```python
from build123d import *

# Parameters (mm, degrees)
F0_W         = 152.4
F0_H         = 44.45
F1_DEPTH     = 2
F2_W         = 152.4
F2_H         = 6.35
F3_DEPTH     = 18.796
F4_R         = 1.75
F5_DEPTH     = 25
F7_DEPTH     = 25.401
F8_SIZE      = 1.8
F9_T4_DEPTH  = 152.4
F9_S5_R      = 9
F9_T6_DEPTH  = 78
F9_T10_DEPTH = 152.4
F9_S11_R     = 9
F9_T12_DEPTH = 78
F10_R        = 2


# Not quite as in the source:
# - a fillet or chamfer that OpenCascade refuses, or shapes differently, is made with other operations: its cross-section is extruded or revolved along the edge and cut away or added
# - a feature names something its author has since deleted; it is built from what else it names


with BuildPart() as f1:
    # F0 (on Top) → F1 (new body)
    with BuildSketch(Plane.XY):
        Rectangle(F0_W, F0_H)
    extrude(amount=F1_DEPTH)

    # F2 (on face) → F3 (join)
    with BuildSketch(Plane(origin=(0, 0, 0), x_dir=(1, 0, 0), z_dir=(0, 0, -1))):
        Rectangle(F2_W, F2_H)
    extrude(amount=F3_DEPTH)

    # F4 (on face) → F5 (cut)
    with BuildSketch(Plane(origin=(0, 0, 0), x_dir=(1, 0, 0), z_dir=(0, 0, -1))):
        with Locations((48, -12.7)):
            Circle(F4_R)
        with Locations((-48, -12.7)):
            Circle(F4_R)
        with Locations((-48, 12.7)):
            Circle(F4_R)
        with Locations((48, 12.7)):
            Circle(F4_R)
    extrude(amount=-F5_DEPTH, mode=Mode.SUBTRACT)

    # F6 (on face) → F7 (cut, through all)
    with BuildSketch(Plane(origin=(0, 3.175, 0), x_dir=(-1, 0, 0), z_dir=(0, 1, 0))):
        with BuildLine():
            ThreePointArc((-9, -9.398), (0, -18.398), (9, -9.398))
            ThreePointArc((9, -9.398), (0, -0.398), (-9, -9.398))
        make_face()
        with BuildLine():
            Line((9, -18.796), (9, -9.398))
            ThreePointArc((9, -9.398), (0, -18.398), (-9, -9.398))
            Line((-9, -9.398), (-9, -18.796))
            Line((-9, -18.796), (9, -18.796))
        make_face()
    extrude(amount=-F7_DEPTH, mode=Mode.SUBTRACT)

    # F8
    f8_edges = [f1.edges().sort_by_distance(p)[0] for p in [
        (46.25, -12.7, 2),
        (-49.75, -12.7, 2),
        (-49.75, 12.7, 2),
        (46.25, 12.7, 2),
    ]]
    chamfer(f8_edges, length=F8_SIZE)

    # F9: chamfer of 1 on 2 edges, made by hand


with BuildPart() as f9_tool2:
    # F9_s3 → F9_t4 (new body)
    with BuildSketch(Plane.YZ.offset(-76.2)):
        Polygon((3.175, -1), (4.175, 0), (3.175, 0), align=None)
    extrude(amount=F9_T4_DEPTH)

    # F9_s5 → F9_t6 (cut, symmetric)
    with BuildSketch(Plane.XZ.offset(-3.7)):
        with Locations((0, -9.398)):
            Circle(F9_S5_R)
    extrude(amount=F9_T6_DEPTH, both=True, mode=Mode.SUBTRACT)


with BuildPart() as f1_1:
    add(f1.part)

    # F9_t1: union F9_tool2
    add(f9_tool2.part)


with BuildPart() as f9_tool8:
    # F9_s9 → F9_t10 (new body)
    with BuildSketch(Plane.YZ.offset(76.2)):
        Polygon((-4.175, 0), (-3.175, -1), (-3.175, 0), align=None)
    extrude(amount=-F9_T10_DEPTH)

    # F9_s11 → F9_t12 (cut, symmetric)
    with BuildSketch(Plane.XZ.offset(3.7)):
        with Locations((0, -9.398)):
            Circle(F9_S11_R)
    extrude(amount=F9_T12_DEPTH, both=True, mode=Mode.SUBTRACT)


with BuildPart() as f1_2:
    add(f1_1.part)

    # F9_t7: union F9_tool8
    add(f9_tool8.part)

    # F10
    f10_edges = [f1_2.edges().sort_by_distance(p)[0] for p in [
        (9, 0, -18.796),
        (-9, 0, -18.796),
    ]]
    fillet(f10_edges, radius=F10_R)


solid = f1_2.part
```
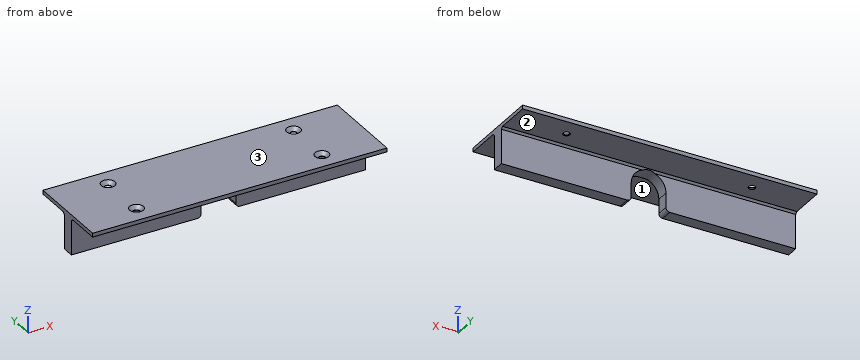
The model under review builds one solid part; all positions refer to its coordinate system, in mm. Face numbers are marked on the shaded views. A direction names the side the tool comes from. Coordinates: 2 decimals unless noted, no trailing zeros. Loops run counter-clockwise (first coordinate to the right, second up) from the corner with the lowest first, then second, coordinate; pieces in that order, holes last. Notation, with made-up numbers: (59, 61) -> (79, 61) arc R18 ccw to (79, 83) -> close; hole circle Ø6 at (70, 70). An arc over 180 degrees is marked (long way). Answer as CSV lines item,"result".
Item 1: Take a section at B-B, the plane z = -12.75. State the section outline as (x, y) points (3 decimals).
Results below:
outline,"(-76.2, -3.175) -> (-9, -3.175) -> (-9, 3.175) -> (-76.2, 3.175) -> close; (9, -3.175) -> (76.2, -3.175) -> (76.2, 3.175) -> (9, 3.175) -> close"
Item 2: Take a section at D-D, the plane x = 0. State the section outline as (y, z) points (3 decimals).
Results below:
outline,"(-22.225, 0) -> (-4.175, 0) -> (-3.777, -0.398) -> (3.777, -0.398) -> (4.175, 0) -> (22.225, 0) -> (22.225, 2) -> (-22.225, 2) -> close"
Item 3: Take a section at A-A, the plane x = 48. State the section outline as (y, z) points (3 decimals), and give its area (3 significant figures).
Results below:
outline,"(-22.225, 0) -> (-14.45, 0) -> (-14.45, 0.2) -> (-16.25, 2) -> (-22.225, 2) -> close; (-10.95, 0) -> (-4.175, 0) -> (-3.175, -1) -> (-3.175, -18.796) -> (3.175, -18.796) -> (3.175, -1) -> (4.175, 0) -> (10.95, 0) -> (10.95, 0.2) -> (9.15, 2) -> (-9.15, 2) -> (-10.95, 0.2) -> close; (14.45, 0) -> (22.225, 0) -> (22.225, 2) -> (16.25, 2) -> (14.45, 0.2) -> close"
area,"189 mm2"
Item 4: Insertion check: pin 1 (12 mm diameter, centred on x = -13, z = -11.5, fed in from -Y) (3 decimals); pin 2 (10 mm diameter, centred on x = -16.5, z = -7.5, fed in from +Y) (3 decimals); pin 3 (3 mm diameter, centred on x = -48, y = 12.7, fed in from -Z); pin 4 (5.5 mm diameter, centred on x = 17, y = 13.5, fed in from -Z). Each pin has a flat end and moves straight along its axis. Give the tip position at first contact, or say it passes through.
Results below:
pin 1,"stops at y = -3.175"
pin 2,"stops at y = 3.175"
pin 3,"passes through"
pin 4,"stops at z = 0"
Item 5: Machinability: for the marked faces 1, 2 and 3, which of the approach directions +Z, -Z, +X, -X, +Y, -Y give a long, thin tool a straight path to every point of the face, cutting with its end or side? Answer none if there is none.
Results below:
face 1,"-Z, +X, -X, -Y"
face 2,"-Z, +X, -X, +Y"
face 3,"+Z, +X, -X, +Y, -Y"
Item 6: Take a section at C-C, the plane y = 12.7. State the section outline as (x, z) points.
Results below:
outline,"(-76.2, 0) -> (-49.75, 0) -> (-49.75, 0.2) -> (-51.55, 2) -> (-76.2, 2) -> close; (-46.25, 0) -> (46.25, 0) -> (46.25, 0.2) -> (44.45, 2) -> (-44.45, 2) -> (-46.25, 0.2) -> close; (49.75, 0) -> (76.2, 0) -> (76.2, 2) -> (51.55, 2) -> (49.75, 0.2) -> close"
Item 7: For L1, parallel to Y at x = 48, z = 0.1 (3 decimals); L2, parallel to X at y = -12.7, z = 0.1; L3, parallel to Z at x = -6, y = 7, list the stretches that pass through material, from the lowest coordinate up.
Results below:
L1,"y = -22.225 to -14.45, -10.95 to 10.95, 14.45 to 22.225"
L2,"x = -76.2 to -49.75, -46.25 to 46.25, 49.75 to 76.2"
L3,"z = 0 to 2"
